Geometry: final body of the model. Coordinates: model frame, mm. Give positions to 0.01 mm unless a question says otherwise; leave off trailing zeros. Order: outer loops, then holes, each group sorted by start corner. A loop starts at its lowest first (then second) coordinate and runs counter-clockwise, first axis right, second up. Notation, with made-up numbers: (-7.5, 60) -> (38.5, 60) arc R18 cw to (38.5, 74) -> close; hole circle Ø6 at (-14.75, 76). An arc over 180 degrees is marked (long way). Write item = value, one per line.
```python
from build123d import *

# Parameters (mm, degrees)
F0_W       = 152.4
F0_H       = 152.4
F1_DEPTH   = 152.4
F2_SIZE    = 5
F3_R       = 36.5
F4_DEPTH   = 152.401
F7_D       = 73
F7_ON_F5_D = 73


with BuildPart() as f1:
    # F0 (on Front) → F1 (new body)
    with BuildSketch(Plane.XZ):
        Rectangle(F0_W, F0_H)
    extrude(amount=F1_DEPTH)

    # F2
    f2_edges = [f1.edges().sort_by_distance(p)[0] for p in [
        (0, -152.4, 76.2),
        (-76.2, -76.2, 76.2),
        (76.2, -76.2, 76.2),
        (0, 0, 76.2),
        (76.2, -152.4, 0),
        (-76.2, -152.4, 0),
        (0, -152.4, -76.2),
        (76.2, -76.2, -76.2),
        (76.2, 0, 0),
        (-76.2, 0, 0),
        (0, 0, -76.2),
        (-76.2, -76.2, -76.2),
    ]]
    chamfer(f2_edges, length=F2_SIZE)

    # F3 (on face) → F4 (cut, through all)
    with BuildSketch(Plane(origin=(0, 0, 0), x_dir=(-1, 0, 0), z_dir=(0, 1, 0))):
        Circle(F3_R)
    extrude(amount=-F4_DEPTH, mode=Mode.SUBTRACT)

    # F7 (through all)
    with Locations(Plane(origin=(-76.2, 0, 0), x_dir=(0, -1, 0), z_dir=(-1, 0, 0))):
        with Locations((76.2, 0)):
            Hole(F7_D / 2)

    # F7 on F5 (through all)
    with Locations(Plane(origin=(0, 0, -76.2), x_dir=(1, 0, 0), z_dir=(0, 0, -1))):
        with Locations((0, 76.2)):
            Hole(F7_ON_F5_D / 2)


solid = f1.part
```
1) Section query C-C (x = 51.5). Output: boundary loops of the cut face in (y, z), plus the area to 3 significant figures.
Check sheet entries:
outline = (-152.4, -71.2) -> (-147.4, -76.2) -> (-5, -76.2) -> (0, -71.2) -> (0, 71.2) -> (-5, 76.2) -> (-147.4, 76.2) -> (-152.4, 71.2) -> close; hole circle Ø73 at (-76.2, 0)
area = 19,000 mm²
2) Section query A-A (y = -76.2). Output: boundary loops of the cut face in (x, z), plus the area to 3 significant figures.
Check sheet entries:
outline = (-76.2, -71.2) -> (-71.2, -76.2) -> (-36.5, -76.2) -> (-36.5, -36.5) -> (-76.2, -36.5) -> close; (-76.2, 36.5) -> (-36.5, 36.5) -> (-36.5, 76.2) -> (-71.2, 76.2) -> (-76.2, 71.2) -> close; (36.5, -76.2) -> (71.2, -76.2) -> (76.2, -71.2) -> (76.2, -36.5) -> (36.5, -36.5) -> close; (36.5, 36.5) -> (76.2, 36.5) -> (76.2, 71.2) -> (71.2, 76.2) -> (36.5, 76.2) -> close
area = 6,250 mm²
3) First-contact query: P1, Ø4, axis at x = -16, y = -107.5, coming from the +Z side. Flat tip, straight axial feed; report the tip coordinate or a pass-through.
Check sheet entries:
P1 = 76.2
4) Mould query, pull axis Z, two halves, no side actions, for faces 1 (the face through (-73.7, -75.2, 73.7)), 2 (the face through (-17, 0, 33)), 3 (the face through (26.9, -19.24, 24.67)), 4 (the face through (-1, -2.5, -73.7)). Classes: +Z half, -Z half, draft (parallel to the pull), parting line (faces both ways), or undercut.
Check sheet entries:
face_1 = +Z half
face_2 = draft
face_3 = undercut
face_4 = -Z half
5) Line query: line 1 (Y direction, x = 0, z = 64.5); line 2 (X direction, y = -21.5, z = 0). Output: solid intervals per line, ascending. Write a range as from..to.
Check sheet entries:
line_1 = -152.4..-112.7, -39.7..0
line_2 = -76.2..-36.5, 36.5..76.2
6) Section query B-B (z = 0). Output: boundary loops of the cut face in (x, y), plus the area to 3 significant figures.
Check sheet entries:
outline = (-76.2, -147.4) -> (-71.2, -152.4) -> (-36.5, -152.4) -> (-36.5, -112.7) -> (-76.2, -112.7) -> close; (-76.2, -39.7) -> (-36.5, -39.7) -> (-36.5, 0) -> (-71.2, 0) -> (-76.2, -5) -> close; (36.5, -152.4) -> (71.2, -152.4) -> (76.2, -147.4) -> (76.2, -112.7) -> (36.5, -112.7) -> close; (36.5, -39.7) -> (76.2, -39.7) -> (76.2, -5) -> (71.2, 0) -> (36.5, 0) -> close
area = 6,250 mm²
7) Section query D-D (y = -126). Output: boundary loops of the cut face in (x, z), plus the area to 3 significant figures.
Check sheet entries:
outline = (-76.2, -71.2) -> (-71.2, -76.2) -> (71.2, -76.2) -> (76.2, -71.2) -> (76.2, 71.2) -> (71.2, 76.2) -> (-71.2, 76.2) -> (-76.2, 71.2) -> close; hole circle Ø73 at (0, 0)
area = 19,000 mm²
